from build123d import *

# Parameters (mm, degrees)
SKETCH2_R           = 3
SKETCH2_R_2         = 1
BOSS_EXTRUDE1_DEPTH = 6
SKETCH3_R           = 1.5
BOSS_EXTRUDE2_DEPTH = 1.7


with BuildPart() as part:
    # Sketch2 → Boss-Extrude1 (new body)
    with BuildSketch(Plane(origin=(0, 0, 0), x_dir=(1, 0, 0), z_dir=(0, 1, 0))):
        with Locations(Location((0, 0, 0), (0, 0, 270))):
            Circle(SKETCH2_R)
        with Locations(Location((0, 0, 0), (0, 0, 270))):
            Circle(SKETCH2_R_2, mode=Mode.SUBTRACT)
    extrude(amount=BOSS_EXTRUDE1_DEPTH)

    # Sketch3 → Boss-Extrude2 (add)
    with BuildSketch(Plane(origin=(0, 6, 0), x_dir=(1, 0, 0), z_dir=(0, 1, 0))):
        with Locations(Location((0, 0, 0), (0, 0, 270))):
            Circle(SKETCH3_R)
    extrude(amount=BOSS_EXTRUDE2_DEPTH)


solid = part.part
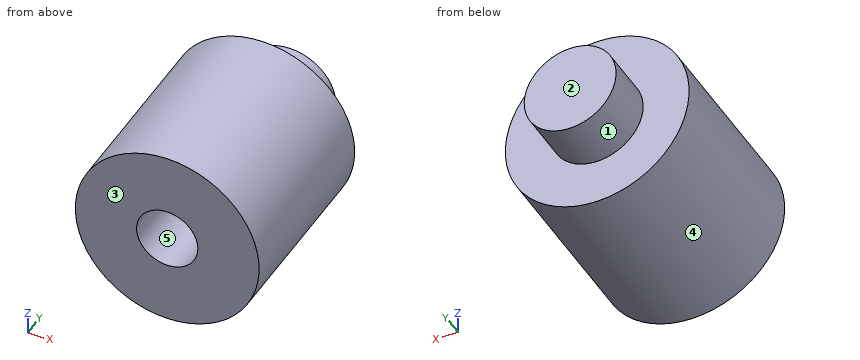
Build history of the part. All positions in model axes, mm. Face numbers are marked on the shaded views. A direction names the side the tool comes from. Round coordinates to 2 decimals unless told otherwise and drop trailing zeros. Write each loop counter-clockwise with the first axis right and the second up, starting at its lowest first coordinate (ties: lowest second). Pieces come first, ordered by that corner, then holes. Notation, with made-up numbers: (47.5, -29) - (75.5, -29) arc R14 ccw to (75.5, -13) - close; hole circle Ø6 at (-35.75, 1.25). An arc over 180 degrees is marked (long way). One line per question, with ' | ' between items.
1. Band-saw the part on C-C, the plane y = 1.5. Write the cut outline in (x, z), and give its area (3 significant figures).
Results are:
outline: circle Ø6 at (0, 0); hole circle Ø2 at (0, 0) | area: 25.1 mm^2
2. Band-saw the part on B-B, the plane x = 0. Write the cut outline in (y, z), and give its area (3 significant figures).
Results are:
outline: (0, -3) - (6, -3) - (6, -1.5) - (7.7, -1.5) - (7.7, 1.5) - (6, 1.5) - (6, 3) - (0, 3) - (0, 1) - (6, 1) - (6, -1) - (0, -1) - close | area: 29.1 mm^2
3. Tool access for the marked faces 1 and 2: list every direction of +Z, -Z, +X, -X, +Y, -Y with a clear straight run to the whole face (end or side of a thin tool).
Results are:
face 1: +Y | face 2: +Z, -Z, +X, -X, +Y
4. Band-saw the part on A-A, the plane z = 0. Write the cut outline in (x, y).
Results are:
outline: (-3, 0) - (-1, 0) - (-1, 6) - (1, 6) - (1, 0) - (3, 0) - (3, 6) - (1.5, 6) - (1.5, 7.7) - (-1.5, 7.7) - (-1.5, 6) - (-3, 6) - close
5. Band-saw the part on D-D, the plane y = 7. Write the cut outline in (x, z).
Results are:
outline: circle Ø3 at (0, 0)
6. Drill centre lines: line 1 along X through (y, z) = (3.8, 0); line 2 along Y through (x, z) = (-2.2, -0.05); line 3 along Z through (x, y) = (-0.65, 2.5). Where is each one in solid material? Low to high. Write a range as from..to.
Results are:
line 1: -3..-1, 1..3 | line 2: 0..6 | line 3: -2.93..-0.76, 0.76..2.93
7. Mould opens along Z. For the marked faces 3, 4 and 5 say: released by +Z, released by -Z, zero draft, split by the parting line, or undercut.
Results are:
face 3: zero draft | face 4: split by the parting line | face 5: undercut
8. Drop flat-ended pins along their axis: pin 1 Ø2 at (x, z) = (0.5, 0.5) entering from -Y; pin 2 Ø2 at (y, z) = (6, 2) entering from +X; pin 3 Ø1.5 at (x, z) = (2, -2) entering from +Y. Give the stop position or say it passes through.
Results are:
pin 1: y = 0 | pin 2: x = 2.83 | pin 3: y = 6
